Read the model definition and answer for the solid it produces. Units are mm, in the model's axes. A direction names the side the tool comes from. Round coordinates to 2 decimals unless told otherwise and drop trailing zeros. Order: outer loops, then holes, each group sorted by start corner. A loop starts at its lowest first (then second) coordinate and runs counter-clockwise, first axis right, second up. Notation, with made-up numbers: (57, 85) - (81, 85) arc R26 cw to (81, 107) - close; hole circle Ø7 at (60.25, 80). An arc over 180 degrees is marked (long way). One line per question, with ' | ' between items. Start each with the question number.
1) The mould has two halves that part along Z. Classify faces 4 (the flat face through (1, -41.317, -10)), 5 (the flat face through (1, -33, -13.442)), 6 (the flat face through (1, -38.317, 1)), 7 (the flat face through (1, 36, -6.067)): pulls with the +Z half, pulls with the -Z half, needs draft (parallel to the pull), parting line crosses it, or undercut.
2) Flat-ended cylindrical pins translate along their axes: pin 1 (1.5 mm diameter, centred on x = 1.5, z = 20.5, fed in from -Y); pin 2 (6 mm diameter, centred on y = 28.5, z = -4.5, fed in from -X); pin 3 (0.9 mm diameter, centred on x = 2, y = -40, fed in from +Z); pin 4 (0.9 mm diameter, centred on x = 1, y = 12.5, fed in from -Z). Find the tip coordinate at first contact, or state that the pin passes through.
3) Straight lines are drawn through the part: line 1 (Y direction, x = 1.35, z = -7.5); line 2 (Z direction, x = 0.6, y = 26.5); line 3 (Y direction, x = 1.5, z = -15). For each, find the intervals that lie inside material, in ascending order. Write a range as from..to.
4) The part is cut by section C-C, the plane y = 9.5. Give the vertices of the cut face in (x, z), plus the area to 3 significant figures.
5) The part is cut by section A-A, the plane z = -10. Give the vertices of the cut face in (x, y), plus the area to 3 significant figures.
6) The part is cut by section D-D, the plane z = -2.5. Give the vertices of the cut face in (x, y), plus the area to 3 significant figures.
7) For faces 1 (the flat face through (1, 4.958, 20)), 2 (the flat face through (1, 28, -13.442)), 3 (the flat face through (1, 19.208, 20)), determine the directions among +Z, -Z, +X, -X, +Y, -Y from which every point of the face is accessible in a straight line to the end or side of a thin tool.
from build123d import *

# Parameters (mm, degrees)
BOSS_EXTRUDE1_DEPTH = 3
SKETCH2_W           = 11
SKETCH2_H           = 11.192112216
CUT_EXTRUDE1_DEPTH  = 10


with BuildPart() as part:
    # Sketch1 → Boss-Extrude1 (new body)
    with BuildSketch(Plane(origin=(0, 0, 0), x_dir=(0, 0, -1), z_dir=(1, 0, 0))):
        Polygon((-18.557859796, 36.983092069), (-18.557859796, 19.208092069), (-21.557859796, 19.208092069), (-21.557859796, 4.958092069), (-18.557859796, 4.958092069), (-18.557859796, -9.291907931), (-21.557859796, -9.291907931), (-21.557859796, -23.541907931), (-18.557859796, -23.541907931), (-18.557859796, -37.791907931), (-18.557859796, -41.316907931), (-8.182859796, -41.316907931), (-8.182859796, -38.316907931), (6.067140204, -38.316907931), (6.067140204, -41.316907931), (13.442140204, -41.316907931), (13.442140204, -23.541907931), (16.442140204, -23.541907931), (16.442140204, -9.291907931), (13.442140204, -9.291907931), (13.442140204, 4.958092069), (16.442140204, 4.958092069), (16.442140204, 19.208092069), (13.442140204, 19.208092069), (13.442140204, 33.458092069), (13.442140204, 36.983092069), (6.067140204, 36.983092069), (6.067140204, 33.983092069), (-8.182859796, 33.983092069), (-8.182859796, 36.983092069), align=None)
    extrude(amount=BOSS_EXTRUDE1_DEPTH)

    # Sketch2 → Cut-Extrude1 (cut)
    with BuildSketch(Plane(origin=(3, 0, 0), x_dir=(0, 0, -1), z_dir=(1, 0, 0))):
        with Locations((11.545501323, 10.387035961)):
            Rectangle(SKETCH2_W, SKETCH2_H)
    extrude(amount=-CUT_EXTRUDE1_DEPTH, mode=Mode.SUBTRACT)


solid = part.part
Values:
1) face 4: needs draft | face 5: pulls with the -Z half | face 6: undercut | face 7: undercut
2) pin 1: stops at y = -23.54 | pin 2: stops at x = 0 | pin 3: stops at z = 18.56 | pin 4: stops at z = -6.05
3) line 1: y = -41.32..4.79, 15.98..36.98 | line 2: z = -13.44..18.56 | line 3: y = -23.54..-9.29, 15.98..19.21
4) outline: (0, -6.05) - (3, -6.05) - (3, 21.56) - (0, 21.56) - close | area: 82.8 mm^2
5) outline: (0, -41.32) - (3, -41.32) - (3, 4.79) - (0, 4.79) - close; (0, 15.98) - (3, 15.98) - (3, 36.98) - (0, 36.98) - close | area: 201 mm^2
6) outline: (0, -38.32) - (3, -38.32) - (3, 33.98) - (0, 33.98) - close | area: 217 mm^2
7) face 1: +Z, +X, -X | face 2: -Z, +X, -X, +Y | face 3: +Z, +X, -X, +Y
